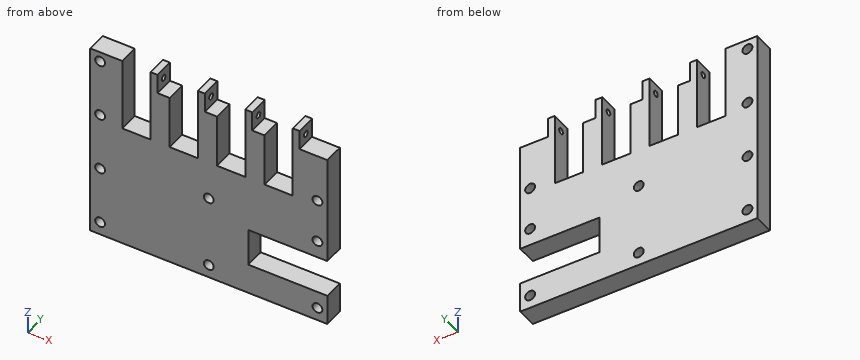
```python
from build123d import *

# Parameters (mm, degrees)
SKETCH1_W                 = 120
SKETCH1_H                 = 100
BOSS_EXTRUDE1_DEPTH       = 10
CUT_EXTRUDE1_DEPTH        = 37
SKETCH3_W                 = 6.2125
SKETCH3_H                 = 10
SKETCH3_W_2               = 14
CUT_EXTRUDE2_DEPTH        = 10
SKETCH4_R                 = 1.5
CUT_EXTRUDE3_DEPTH        = 75.5
SKETCH7_R                 = 2.5
SKETCH7_W                 = 40
SKETCH7_H                 = 19.05
CUT_EXTRUDE4_DEPTH        = 20
SKETCH10_R                = 2.5
CUT_EXTRUDE5_DEPTH        = 10
F_5_0MM_DOWEL_HOLE1_D     = 5
F_5_0MM_DOWEL_HOLE1_DEPTH = 25
F_5_0MM_DOWEL_HOLE1_TIP   = 1.502151548


with BuildPart() as part:
    # Sketch1 → Boss-Extrude1 (new body)
    with BuildSketch(Plane(origin=(0, 0, 0), x_dir=(1, 0, 0), z_dir=(0, 1, 0))):
        Rectangle(SKETCH1_W, SKETCH1_H)
    extrude(amount=BOSS_EXTRUDE1_DEPTH)

    # Sketch2 → Cut-Extrude1 (cut)
    with BuildSketch(Plane.XY.offset(50)):
        Polygon((-42.5, 10), (-43.7875, 10), (-43.7875, -10), (-42.5, -10), (-29.5, -10), (-29.5, 10), align=None)
        Polygon((-5.5, -10), (-18.5, -10), (-19.7875, -10), (-19.7875, 10), (-18.5, 10), (-5.5, 10), align=None)
        Polygon((18.5, -10), (5.5, -10), (4.2125, -10), (4.2125, 10), (5.5, 10), (18.5, 10), align=None)
        Polygon((42.5, -10), (29.5, -10), (28.2125, -10), (28.2125, 10), (29.5, 10), (42.5, 10), align=None)
    extrude(amount=-CUT_EXTRUDE1_DEPTH, mode=Mode.SUBTRACT)

    # Sketch3 → Cut-Extrude2 (cut)
    with BuildSketch(Plane.XY.offset(50)):
        with Locations((-22.89375, 5)):
            Rectangle(SKETCH3_W, SKETCH3_H)
        with Locations((1.10625, 5)):
            Rectangle(SKETCH3_W, SKETCH3_H)
        with Locations((25.10625, 5)):
            Rectangle(SKETCH3_W, SKETCH3_H)
        with Locations((53, 5)):
            Rectangle(SKETCH3_W_2, SKETCH3_H)
    extrude(amount=-CUT_EXTRUDE2_DEPTH, mode=Mode.SUBTRACT)

    # Sketch4 → Cut-Extrude3 (cut)
    with BuildSketch(Plane(origin=(46, 0, 0), x_dir=(0, 0, -1), z_dir=(1, 0, 0))):
        with Locations((-45, 5)):
            Circle(SKETCH4_R)
    extrude(amount=-CUT_EXTRUDE3_DEPTH, mode=Mode.SUBTRACT)

    # Sketch7 → Cut-Extrude4 (cut)
    with BuildSketch(Plane(origin=(0, 10, 0), x_dir=(1, 0, 0), z_dir=(0, 1, 0))):
        with Locations((55, 6.7125)):
            Circle(SKETCH7_R)
        with Locations((55, 43.2875)):
            Circle(SKETCH7_R)
        with Locations((0, 43.2875)):
            Circle(SKETCH7_R)
        with Locations((0, 6.7125)):
            Circle(SKETCH7_R)
        with Locations((40, 25)):
            Rectangle(SKETCH7_W, SKETCH7_H)
    extrude(amount=-CUT_EXTRUDE4_DEPTH, mode=Mode.SUBTRACT)

    # Sketch10 → Cut-Extrude5 (cut)
    with BuildSketch(Plane(origin=(0, 10, 0), x_dir=(1, 0, 0), z_dir=(0, 1, 0))):
        with Locations((-55, 43.2875)):
            Circle(SKETCH10_R)
        with Locations((55, 43.2875)):
            Circle(SKETCH10_R)
        with Locations((55, 6.7125)):
            Circle(SKETCH10_R)
        with Locations((-55, 13.858333333)):
            Circle(SKETCH10_R)
        with Locations((-55, -15.570833333)):
            Circle(SKETCH10_R)
        with Locations((-55, -45)):
            Circle(SKETCH10_R)
        with Locations((55, -15.570833333)):
            Circle(SKETCH10_R)
    extrude(amount=-CUT_EXTRUDE5_DEPTH, mode=Mode.SUBTRACT)

    # Ø5.0mm Dowel Hole1
    with Locations(Plane(origin=(-676.293536786, 10, -1303.282701689), x_dir=(1, 0, 0), z_dir=(0, 1, 0))):
        with Locations((731.293536786, -1318.853535022), (621.293536786, -1318.853535022), (621.293536786, -1348.282701689), (621.293536786, -1259.995201689), (731.293536786, -1259.995201689), (731.293536786, -1296.570201689), (621.293536786, -1289.424368355)):
            Hole(F_5_0MM_DOWEL_HOLE1_D / 2, depth=F_5_0MM_DOWEL_HOLE1_DEPTH)
            with Locations((0, 0, -(F_5_0MM_DOWEL_HOLE1_DEPTH + F_5_0MM_DOWEL_HOLE1_TIP / 2))):  # 118° drill point
                Cone(0, F_5_0MM_DOWEL_HOLE1_D / 2, F_5_0MM_DOWEL_HOLE1_TIP, mode=Mode.SUBTRACT)


solid = part.part
```
Check sheet for the modelled part. Datum: model origin and axes. Units: mm. Coordinates: 2 decimals unless noted, no trailing zeros. Loops run counter-clockwise (first coordinate to the right, second up) from the corner with the lowest first, then second, coordinate; pieces in that order, holes last.
1) Material ranges on probe 1 along Z at (x, y) = (-55, 7.5); probe 2 along Z at (x, y) = (55, 6.5) (1 decimal); probe 3 along X at (y, z) = (5.5, -43), recorded low to high.
2) Sectioned sample at A-A (x = -55). Record the boundary of the cut face in (y, z), and give its area (3 significant figures).
3) Sectioned sample at B-B (z = 36). Record the boundary of the cut face in (x, y).
4) Gauge pin test, flat ends, axial feed: pin 1 (4 mm diameter, centred on x = -55, z = -13.86, fed in from +Y); pin 2 (6 mm diameter, centred on x = 55, z = -6.71, fed in from +Y); pin 3 (2 mm diameter, centred on x = 1, y = 2.5, fed in from +Z); pin 4 (4 mm diameter, centred on x = -16.5, y = 3.5, fed in from +Z). Record the tip position at first contact, or that the pin passes through.
5) Sectioned sample at C-C (x = 0). Record the boundary of the cut face in (y, z), and give its area (3 significant figures).
6) Sectioned sample at D-D (y = 5). Count the separate pieces of the cut face and the enclosed holes in it, and give its area (3 significant figures).
Check sheet entries:
1. probe 1: z = -50 to -45.79, -40.79 to -16.36, -11.36 to 13.07, 18.07 to 42.5, 47.5 to 50
1. probe 2: z = -50 to -45.8, -40.8 to -34.5, -15.5 to -9.2, -4.2 to 13.1, 18.1 to 40
1. probe 3: x = -60 to -57.48, -52.52 to -2.48, 2.48 to 52.52, 57.48 to 60
2. outline: (0, -50) - (10, -50) - (10, -45.79) - (0, -45.79) - close; (0, -40.79) - (10, -40.79) - (10, -16.36) - (0, -16.36) - close; (0, -11.36) - (10, -11.36) - (10, 13.07) - (0, 13.07) - close; (0, 18.07) - (10, 18.07) - (10, 42.5) - (0, 42.5) - close; (0, 47.5) - (10, 47.5) - (10, 50) - (0, 50) - close
2. area: 800 mm2
3. outline: (-60, 0) - (-43.79, 0) - (-43.79, 10) - (-60, 10) - close; (-29.5, 0) - (-19.79, 0) - (-19.79, 10) - (-29.5, 10) - close; (-5.5, 0) - (4.21, 0) - (4.21, 10) - (-5.5, 10) - close; (18.5, 0) - (28.21, 0) - (28.21, 10) - (18.5, 10) - close; (42.5, 0) - (60, 0) - (60, 10) - (42.5, 10) - close
4. pin 1: passes through
4. pin 2: stops at y = 10
4. pin 3: stops at z = 40
4. pin 4: stops at z = 13
5. outline: (0, -50) - (10, -50) - (10, -45.79) - (0, -45.79) - close; (0, -40.79) - (10, -40.79) - (10, -9.21) - (0, -9.21) - close; (0, -4.21) - (10, -4.21) - (10, 40) - (0, 40) - close
5. area: 800 mm2
6. separate pieces: 5
6. enclosed holes: 9
6. area: 8,580 mm2
